```python
from build123d import *

# Parameters (mm, degrees)
SKETCH1_W           = 25
SKETCH1_H           = 23
BOSS_EXTRUDE1_DEPTH = 15
BOSS_EXTRUDE4_DEPTH = 5
SKETCH3_R           = 1.55
BOSS_EXTRUDE5_DEPTH = 5
SKETCH1_6_W         = 25
SKETCH1_6_H         = 2
BOSS_EXTRUDE6_DEPTH = 25


with BuildPart() as part:
    # Sketch1 → Boss-Extrude1 (new body)
    with BuildSketch(Plane.XY):
        with Locations((0, -1)):
            Rectangle(SKETCH1_W, SKETCH1_H)
        with BuildLine():
            Line((8.5, -2.5), (8.5, -4.5))
            Line((8.5, -4.5), (1.118033989, -4.5))
            ThreePointArc((1.118033989, -4.5), (0, -5), (-1.118033989, -4.5))
            Line((-1.118033989, -4.5), (-8.5, -4.5))
            Line((-8.5, -4.5), (-8.5, -2.5))
            Line((-8.5, -2.5), (-1.118033989, -2.5))
            ThreePointArc((-1.118033989, -2.5), (0, -2), (1.118033989, -2.5))
            Line((1.118033989, -2.5), (8.5, -2.5))
        make_face(mode=Mode.SUBTRACT)
        with BuildLine():
            Line((8.5, 9.5), (8.5, 7.5))
            Line((8.5, 7.5), (1.118033989, 7.5))
            ThreePointArc((1.118033989, 7.5), (0, 7), (-1.118033989, 7.5))
            Line((-1.118033989, 7.5), (-8.5, 7.5))
            Line((-8.5, 7.5), (-8.5, 9.5))
            Line((-8.5, 9.5), (-1.118033989, 9.5))
            ThreePointArc((-1.118033989, 9.5), (0, 10), (1.118033989, 9.5))
            Line((1.118033989, 9.5), (8.5, 9.5))
        make_face(mode=Mode.SUBTRACT)
    extrude(amount=BOSS_EXTRUDE1_DEPTH)

    # Sketch1_5 → Boss-Extrude4 (add)
    with BuildSketch(Plane.XY):
        with BuildLine():
            Line((-8.5, 7.5), (-1.118033989, 7.5))
            ThreePointArc((-1.118033989, 7.5), (-1.5, 8.5), (-1.118033989, 9.5))
            Line((-1.118033989, 9.5), (-8.5, 9.5))
            Line((-8.5, 9.5), (-8.5, 7.5))
        make_face()
        with BuildLine():
            Line((1.118033989, 7.5), (8.5, 7.5))
            Line((8.5, 7.5), (8.5, 9.5))
            Line((8.5, 9.5), (1.118033989, 9.5))
            ThreePointArc((1.118033989, 9.5), (1.401258538, 9.035233135), (1.5, 8.5))
            ThreePointArc((1.5, 8.5), (1.401258538, 7.964766865), (1.118033989, 7.5))
        make_face()
        with BuildLine():
            Line((1.118033989, -4.5), (8.5, -4.5))
            Line((8.5, -4.5), (8.5, -2.5))
            Line((8.5, -2.5), (1.118033989, -2.5))
            ThreePointArc((1.118033989, -2.5), (1.401258538, -2.964766865), (1.5, -3.5))
            ThreePointArc((1.5, -3.5), (1.401258538, -4.035233135), (1.118033989, -4.5))
        make_face()
        with BuildLine():
            Line((-8.5, -4.5), (-1.118033989, -4.5))
            ThreePointArc((-1.118033989, -4.5), (-1.5, -3.5), (-1.118033989, -2.5))
            Line((-1.118033989, -2.5), (-8.5, -2.5))
            Line((-8.5, -2.5), (-8.5, -4.5))
        make_face()
    extrude(amount=BOSS_EXTRUDE4_DEPTH)

    # Sketch3 → Boss-Extrude5 (add)
    with BuildSketch(Plane.XZ.offset(12.5)):
        with BuildLine():
            Line((-12.5, 15), (-17.125197634, 12.142130014))
            ThreePointArc((-17.125197634, 12.142130014), (-18.168457468, 11.051043611), (-18.548267571, 9.590014896))
            Line((-18.548267571, 9.590014896), (-18.548267571, 5.461294281))
            ThreePointArc((-18.548267571, 5.461294281), (-18.168457468, 4.000265566), (-17.125197634, 2.909179163))
            Line((-17.125197634, 2.909179163), (-12.5, 0.051309177))
            Line((-12.5, 0.051309177), (-12.5, 15))
        make_face()
        with Locations((-15.5, 7.525654589)):
            Circle(SKETCH3_R, mode=Mode.SUBTRACT)
        with BuildLine():
            ThreePointArc((17.125197634, 2.909179163), (18.168457468, 4.000265566), (18.548267571, 5.461294281))
            Line((18.548267571, 5.461294281), (18.548267571, 9.590014896))
            ThreePointArc((18.548267571, 9.590014896), (18.168457468, 11.051043611), (17.125197634, 12.142130014))
            Line((17.125197634, 12.142130014), (12.5, 15))
            Line((12.5, 15), (12.5, 0.051309177))
            Line((12.5, 0.051309177), (17.125197634, 2.909179163))
        make_face()
        with Locations((15.5, 7.525654589)):
            Circle(SKETCH3_R, mode=Mode.SUBTRACT)
    extrude(amount=-BOSS_EXTRUDE5_DEPTH)

    # Sketch1_6 → Boss-Extrude6 (add)
    with BuildSketch(Plane.XY):
        with Locations((0, 11.5)):
            Rectangle(SKETCH1_6_W, SKETCH1_6_H)
    extrude(amount=BOSS_EXTRUDE6_DEPTH)


solid = part.part
```
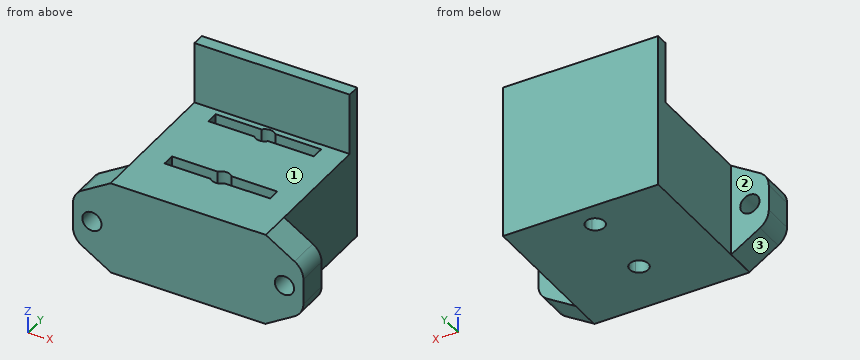
Verification items for the finished model (mm, model axes). Face numbers are marked on the shaded views. A direction names the side the tool comes from. Give positions to 0.01 mm unless a question says otherwise; leave off trailing zeros. Loops run counter-clockwise (first coordinate to the right, second up) from the corner with the lowest first, then second, coordinate; pieces in that order, holes last. Notation, with made-up numbers: M 33,53.25 L 56,53.25 A22 ccw 56,88.25 Z; hole C 75.25,-9 d11. An arc over 180 degrees is marked long. Return JSON: item names as keys, results as strings.
1) Gauge pin test, flat ends, axial feed: P1, Ø1, axis at x = 6, y = -3.5, coming from the +Z side; P2, Ø1.6, axis at y = -3.5, z = 11, coming from the -X side; P3, Ø0.6, axis at y = -3.5, z = 11.5, coming from the +X side. Record the tip position at first contact, or that the pin passes through.
Findings:
{"P1": "stops at z = 5", "P2": "stops at x = -12.5", "P3": "stops at x = 12.5"}
2) Section check D-D, the plane x = -5. Enter the section's corners in (y, z), and give its area (3 significant figures).
Findings:
{"outline": "M -12.5,0 L 12.5,0 L 12.5,25 L 10.5,25 L 10.5,15 L 9.5,15 L 9.5,5 L 7.5,5 L 7.5,15 L -2.5,15 L -2.5,5 L -4.5,5 L -4.5,15 L -12.5,15 Z", "area": "355 mm2"}
3) Section check B-B, the plane y = -10.5. Enter the section's corners in (x, z), and give its area (3 significant figures).
Findings:
{"outline": "M -18.55,5.46 A3 ccw -17.13,2.91 L -12.5,0.05 L -12.5,0 L 12.5,0 L 12.5,0.05 L 17.13,2.91 A3 ccw 18.55,5.46 L 18.55,9.59 A3 ccw 17.13,12.14 L 12.5,15 L -12.5,15 L -17.13,12.14 A3 ccw -18.55,9.59 Z; hole C -15.5,7.53 d3.1; hole C 15.5,7.53 d3.1", "area": "494 mm2"}
4) Tool access check on the marked faces 1, 2 and 3. Record the directions out of +Z, -Z, +X, -X, +Y, -Y that give a thin tool (end or side, any length) a straight path to the whole face; none if there is none.
Findings:
{"face 1": "+Z, +X, -X, -Y", "face 2": "+Z, -Z, -X, +Y", "face 3": "-Z, -X, +Y, -Y"}
5) Section check A-A, the plane x = 0. Enter the section's corners in (y, z).
Findings:
{"outline": "M -12.5,0 L -5,0 L -5,15 L -12.5,15 Z; M -2,0 L 7,0 L 7,15 L -2,15 Z; M 10,0 L 12.5,0 L 12.5,25 L 10.5,25 L 10.5,15 L 10,15 Z"}
6) Section check C-C, the plane x = 15.5. Enter the section's corners in (y, z), and give its area (3 significant figures).
Findings:
{"outline": "M -12.5,1.9 L -7.5,1.9 L -7.5,5.98 L -12.5,5.98 Z; M -12.5,9.08 L -7.5,9.08 L -7.5,13.15 L -12.5,13.15 Z", "area": "40.7 mm2"}
7) Material ranges on L1, parallel to Y at x = -3, z = 9.75; L2, parallel to Y at x = 1, z = 8; L3, parallel to X at y = 8.5, z = 11.25, recorded low to high. Write a range as [from, to].
Findings:
{"L1": "y = [-12.5, -4.5], [-2.5, 7.5], [9.5, 12.5]", "L2": "y = [-12.5, -4.62], [-2.38, 7.38], [9.62, 12.5]", "L3": "x = [-12.5, -8.5], [8.5, 12.5]"}
